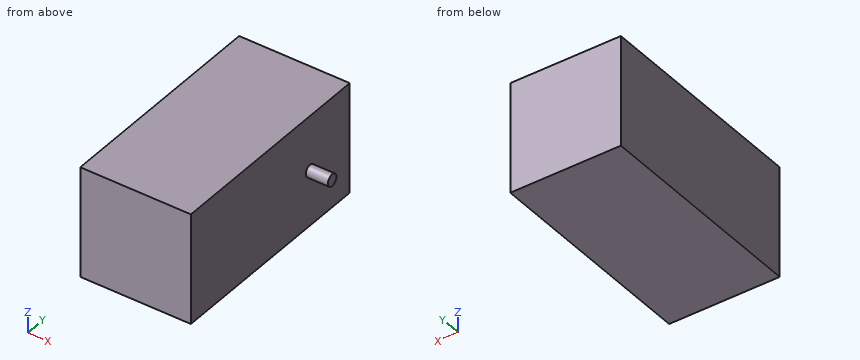
Autodesk Inventor part; units mm, degrees
ref_plane "YZ Plane" through (0, 0, 0) normal (1, 0, 0) x (0, 1, 0)
ref_plane "XZ Plane" through (0, 0, 0) normal (0, 1, 0) x (-1, 0, 0)
ref_plane "XY Plane" through (0, 0, 0) normal (0, 0, 1) x (1, 0, 0)
sketch "Эскиз1" plane through (0, 0, 0) normal (1, 0, 0) x (0, 1, 0)
  line L0 (0, 0) -> (0, -20)
  line L1 (0, -20) -> (40, -20)
  line L2 (40, -20) -> (40, 0)
  line L3 (40, 0) -> (0, 0)
  dimension "d0" = 40
  dimension "d1" = 20
extrude "Выдавливание1" add sketch "Эскиз1" along normal blind 20
sketch "Эскиз2" plane through (20, 0, 0) normal (1, 0, 0) x (0, 0, -1)
  circle A0 centre (10, 30) radius 1.0752
  line L0 (20, 0) -> (20, 40)
  line L1 (20, 40) -> (0, 40)
  point P0 (0, 0)
  dimension "d4" = 10
  dimension "d5" = 10
  dimension "d6" = 2.1503
extrude "Выдавливание2" add sketch "Эскиз2" along normal blind 4
properties part number "мотор"
Could you check a few things on this model? Use its own coordinates, in mm. Round coordinates to 2 decimals unless told otherwise and drop trailing zeros. Order: outer loops, then holes, each group sorted by start corner. A loop starts at its lowest first (then second) coordinate and runs counter-clockwise, first axis right, second up. Notation, with made-up numbers: M 61.5,87.5 L 90.5,87.5 A22 ccw 90.5,120.5 Z; hole C -33.75,75 d5. An arc over 180 degrees is marked long. One line per question, with ' | ' between items. Start each with the question number.
(1) Suppose I cut it at A-A on y = 30. List the corners of the cut face in (x, z) for me, then the cut area to 3 significant figures.
(2) For P1, Ø6, axis at y = 7.5, z = -8.5, coming from the +X side, with a flat end and sliding along its axis, tell me the tip position at first contact or that it passes through.
(3) Please list where these lines run through material, in increasing order: line 1 along X through (y, z) = (18, -8.25); line 2 along Y through (x, z) = (21.5, -10); line 3 along Y through (x, z) = (23, -10.5).
(4) Suppose I cut it at C-C on y = 21. List the corners of the cut face in (x, z) for me.
(5) Suppose I cut it at B-B on z = -10. List the corners of the cut face in (x, y) for me, then the cut area to 3 significant figures.
Geometry results:
1) outline: M 0,-20 L 20,-20 L 20,-11.08 L 24,-11.08 L 24,-8.92 L 20,-8.92 L 20,0 L 0,0 Z | area: 409 mm²
2) P1: x = 20
3) line 1: 0 to 20 | line 2: 28.92 to 31.08 | line 3: 29.05 to 30.95
4) outline: M 0,-20 L 20,-20 L 20,0 L 0,0 Z
5) outline: M 0,0 L 20,0 L 20,28.92 L 24,28.92 L 24,31.08 L 20,31.08 L 20,40 L 0,40 Z | area: 809 mm²
